Input: dimensioned drawing with shaded views. Units: mm. Origin: part minimum x, y, z. A direction names the side the tool comes from. Round coordinates to 2 decimals unless told otherwise and drop trailing zeros. Loops run counter-clockwise (first coordinate to the right, second up) from the corner with the lowest first, then second, coordinate; pieces in that order, holes last. Notation, with made-up numbers: M 17.5,53.5 L 25.5,53.5 A15 cw 25.5,71.5 Z; hole C 58,84.5 d7. An arc over 180 degrees is marked long. One line per item, written item: value.
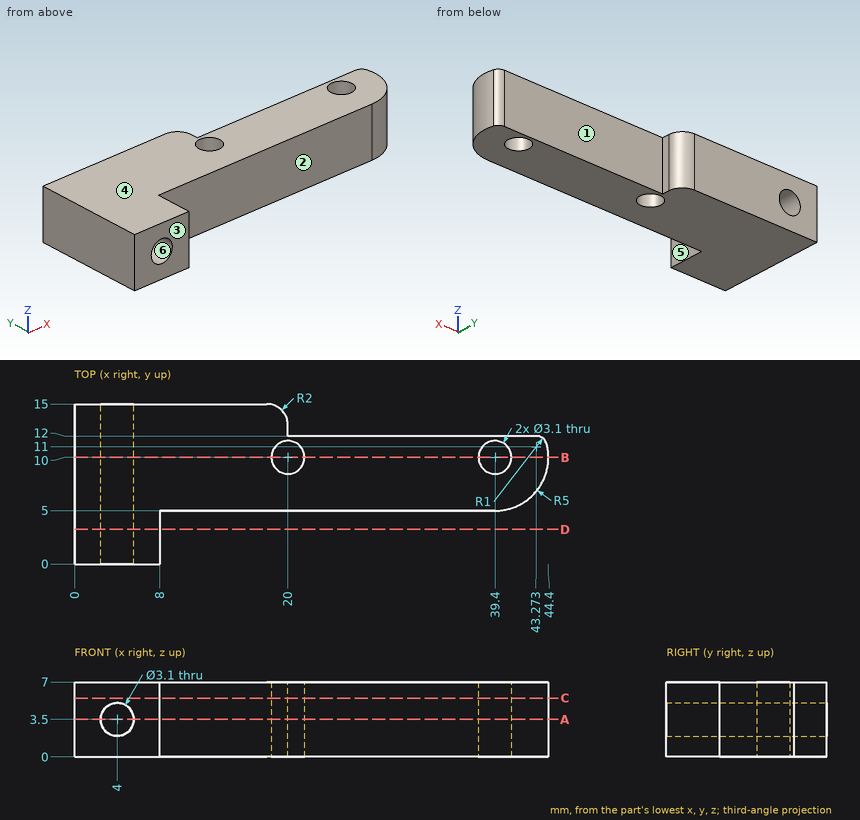
1. Pin query (flat end, axial travel): pin 1 (0.8 mm diameter, centred on y = 12.5, z = 3.5, fed in from +X); pin 2 (2 mm diameter, centred on x = 31.5, z = 2.5, fed in from +Y); pin 3 (1.5 mm diameter, centred on x = 19.5, z = 5.5, fed in from -Y). Return the tip coordinate at first contact, or that it passes through.
Report:
pin 1: stops at x = 20
pin 2: stops at y = 12
pin 3: stops at y = 5
2. Section query C-C (z = 5.5). Return the cut outline in (x, y).
Report:
outline: M 0,0 L 8,0 L 8,5 L 39.4,5 A5 ccw 44.24,11.25 A1 ccw 43.27,12 L 20,12 L 20,13 A2 ccw 18,15 L 0,15 Z; hole C 20,10 d3.1; hole C 39.4,10 d3.1
3. Section query A-A (z = 3.5). Return the cut outline in (x, y).
Report:
outline: M 0,0 L 2.45,0 L 2.45,15 L 0,15 Z; M 5.55,0 L 8,0 L 8,5 L 39.4,5 A5 ccw 44.24,11.25 A1 ccw 43.27,12 L 20,12 L 20,13 A2 ccw 18,15 L 5.55,15 Z; hole C 20,10 d3.1; hole C 39.4,10 d3.1
4. Section query D-D (y = 3.25). Return the cut outline in (x, z), and give its area (3 significant figures).
Report:
outline: M 0,0 L 8,0 L 8,7 L 0,7 Z; hole C 4,3.5 d3.1
area: 48.5 mm2
5. Reachability of the marked faces 1, 2 and 3 from +Z, -Z, +X, -X, +Y, -Y: full face, straight path, thin tool, end or side. Return the list, or none.
Report:
face 1: +Z, -Z, +X, +Y
face 2: +Z, -Z, +X, -Y
face 3: +Z, -Z, +X, -X, -Y
6. Section query B-B (y = 10). Return the cut outline in (x, z), and give its area (3 significant figures).
Report:
outline: M 0,0 L 18.45,0 L 18.45,7 L 0,7 Z; M 21.55,0 L 37.85,0 L 37.85,7 L 21.55,7 Z; M 40.95,0 L 44.4,0 L 44.4,7 L 40.95,7 Z; hole C 4,3.5 d3.1
area: 260 mm2
7. Pull-direction query (Z, two-part tool) for the marked faces 4, 5 and 6; classes: released by +Z, released by -Z, zero draft, split by the parting line, or undercut.
Report:
face 4: released by +Z
face 5: zero draft
face 6: undercut
8. Ray query, line 1 (Z direction, x = 4, y = 5); line 2 (X direction, y = 3.75, z = 3.5); line 3 (Y direction, x = 21, z = 5.25). Return the intervals inside material, ascending. Write a range as [from, to].
Report:
line 1: z = [0, 1.95], [5.05, 7]
line 2: x = [0, 2.45], [5.55, 8]
line 3: y = [5, 8.82], [11.18, 12]
